The model under review builds one solid part; all positions refer to its coordinate system, in mm. A direction names the side the tool comes from. Coordinates: 2 decimals unless noted, no trailing zeros. Loops run counter-clockwise (first coordinate to the right, second up) from the corner with the lowest first, then second, coordinate; pieces in that order, holes last. Notation, with made-up numbers: M 15.25,70.25 L 21.25,70.25 A21 cw 21.25,109.25 Z; hole C 9.5,-37 d3. An arc over 180 degrees is marked long. Use CSV: the item, a comma, the result in double quotes. Start each with the question number.
1. Add section A-A, the plane x = 0. Write out the cut boundary in (y, z).
2. Tool access review of faces 4 (the flat face through (22, 22, -4)), 5 (the flat face through (21, 24, 28)): name each direction out of +Z, -Z, +X, -X, +Y, -Y from which nothing blocks a thin tool from reaching the whole face with its end or side.
3. Clearance check with flat-ended pins moving along their axes: P1, Ø5, axis at x = -17, z = 3, coming from the +Y side; P2, Ø2, axis at y = 12.5, z = 23.5, coming from the +X side; P3, Ø6, axis at x = 21, y = -40, coming from the +Z side; P4, Ø10, axis at x = -38, y = 17.5, coming from the +Z side. State where each tip first meets the part, or that it passes through.
4. For L1, parallel to Y at x = 0, z = 6; L2, parallel to Z at x = -47, y = -0.5, list the stretches that pass through material, from the lowest coordinate up.
5. Add section C-C, the plane z = 19.5. Write out the cut boundary in (x, y).
6. Draft analysis for pull direction Y (two halves, no side actions). For faces 1 (the flat face through (-4.1, 42.3, 28)), 2 (the cylindrical face through (-6.341, 28.554, 11.21)), 3 (the cylindrical face through (28.089, -44.057, 12.224)), state which applies: +Y half, -Y half, draft (parallel to the pull), parting line (faces both ways), or undercut.
from build123d import *

# Parameters (mm, degrees)
F2_R     = 52.25
F2_R_2   = 29.25
F3_DEPTH = 4


with BuildPart() as f1:
    # F0 (on Front) → F1 (revolve)
    with BuildSketch(Plane.XZ):
        with BuildLine():
            Line((40.25, 28), (31.25, 28))
            ThreePointArc((31.25, 28), (29.835786, 27.414214), (29.25, 26))
            Line((29.25, 26), (29.25, 0))
            Line((29.25, 0), (52.25, 0))
            Line((52.25, 0), (52.25, 28))
            Line((52.25, 28), (44.25, 28))
            Line((44.25, 28), (42.25, 28))
            Line((42.25, 28), (41.58282, 29.00077))
            ThreePointArc((41.58282, 29.00077), (41.25, 29.17889), (40.91718, 29.00077))
            Line((40.91718, 29.00077), (40.25, 28))
        make_face()
    revolve(axis=Axis((0, 0, 14), (0, 0, -1)))

    # F2 (on face) → F3 (join)
    with BuildSketch(Plane(origin=(0, 0, 0), x_dir=(1, 0, 0), z_dir=(0, 0, -1))):
        Circle(F2_R)
        Circle(F2_R_2, mode=Mode.SUBTRACT)
    extrude(amount=F3_DEPTH)


solid = f1.part
Computed:
1,outline,"M -52.25,-4 L -29.25,-4 L -29.25,26 A2 ccw -31.25,28 L -40.25,28 L -40.92,29 A0.4 ccw -41.58,29 L -42.25,28 L -52.25,28 Z; M 29.25,-4 L 52.25,-4 L 52.25,28 L 42.25,28 L 41.58,29 A0.4 ccw 40.92,29 L 40.25,28 L 31.25,28 A2 ccw 29.25,26 Z"
2,face 4,"-Z, +X, -X, +Y, -Y"
2,face 5,"+Z"
3,P1,"stops at y = 50.2"
3,P2,"stops at x = 50.97"
3,P3,"stops at z = 28.11"
3,P4,"stops at z = 29.18"
4,L1,"y = -52.25 to -29.25, 29.25 to 52.25"
4,L2,"z = -4 to 28"
5,outline,"C 0,0 d104.5; hole C 0,0 d58.5"
6,face 1,"draft"
6,face 2,"undercut"
6,face 3,"parting line"
